Input: part model. Units: mm. Frame: model coordinates. Round coordinates to 2 decimals unless told otherwise and drop trailing zeros. Loops run counter-clockwise (first coordinate to the right, second up) from the corner with the lowest first, then second, coordinate; pieces in that order, holes last. Notation, with made-up numbers: (61.25, 85.5) - (118.25, 85.5) arc R26 ccw to (118.25, 124.5) - close; hole circle Ø11 at (-26.5, 80). An arc over 180 degrees is marked (long way). Use CSV: the item, a comma, the result in double quotes. Start each with the question number.
1. Cut plane A-A (x = 0.1). Return loops of the section in (y, z).
2. Material intervals for probe 1 along Y at (x, z) = (0.15, -0.75); probe 2 along Y at (x, z) = (-0.2, 5); probe 3 along Z at (x, y) = (0.1, 2), sorted ascending. Write a range as from..to.
3. Cut plane D-D (z = 4.5). Return loops of the section in (x, y), and give its area (3 significant figures).
4. Cut plane B-B (z = 2). Return loops of the section in (x, y), and give its area (3 significant figures).
5. Cut plane C-C (y = 0). Return loops of the section in (x, z).
```python
from build123d import *

# Parameters (mm, degrees)
BOSS_EXTRUDE1_DEPTH      = 0.3175
BOSS_EXTRUDE1_DEPTH_BACK = 0.3175
FILLET1_R                = 0.4445
FILLET2_R                = 0.22225


with BuildPart() as part:
    # Sketch3 → Boss-Extrude1 (new body, two sides)
    with BuildSketch(Plane(origin=(0, 0, 0), x_dir=(0, 0, -1), z_dir=(1, 0, 0))) as boss_extrude1_sk:
        with BuildLine():
            Line((2.493993522, -0.831331174), (4.564354048, -1.521451349))
            ThreePointArc((4.564354048, -1.521451349), (2.8131883, -3.903090272), (0, -4.811251613))
            Line((0, -4.811251613), (0, -2.6289))
            ThreePointArc((0, -2.6289), (-0.831331174, -2.493993522), (-1.57734, -2.10312))
            Line((-1.57734, -2.10312), (-5.759367109, -3.409486899))
            ThreePointArc((-5.759367109, -3.409486899), (6.6929, 0), (-5.759367109, 3.409486899))
            Line((-5.759367109, 3.409486899), (-1.57734, 2.10312))
            ThreePointArc((-1.57734, 2.10312), (-0.831331174, 2.493993522), (0, 2.6289))
            Line((0, 2.6289), (0, 4.811251613))
            ThreePointArc((0, 4.811251613), (2.8131883, 3.903090272), (4.564354048, 1.521451349))
            Line((4.564354048, 1.521451349), (2.493993522, 0.831331174))
            ThreePointArc((2.493993522, 0.831331174), (2.6289, 0), (2.493993522, -0.831331174))
        make_face()
    extrude(amount=BOSS_EXTRUDE1_DEPTH)
    extrude(boss_extrude1_sk.sketch, amount=-BOSS_EXTRUDE1_DEPTH_BACK)

    # Fillet1
    fillet1_edges = [part.edges().sort_by_distance(p)[0] for p in [
        (0, 1.521451349, -4.564354048),
        (0, 4.811251613, 0),
        (0, 3.409486899, 5.759367109),
        (0, -3.409486899, 5.759367109),
        (0, -4.811251613, 0),
        (0, -1.521451349, -4.564354048),
    ]]
    fillet(fillet1_edges, radius=FILLET1_R)

    # Fillet2
    fillet2_edges = [part.edges().sort_by_distance(p)[0] for p in [
        (0, 0.831331174, -2.493993522),
        (0, 2.6289, 0),
        (0, 2.10312, 1.57734),
        (0, -2.10312, 1.57734),
        (0, -2.6289, 0),
        (0, -0.831331174, -2.493993522),
    ]]
    fillet(fillet2_edges, radius=FILLET2_R)


solid = part.part
```
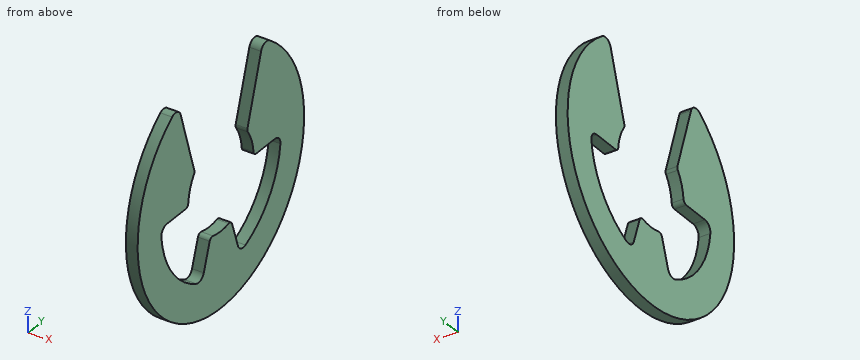
Established:
1,outline,"(-4.79, -0.49) arc R0.44 cw to (-4.34, 0) - (-2.84, 0) arc R0.22 ccw to (-2.62, 0.2) arc R2.63 cw to (-2.17, 1.49) arc R0.22 ccw to (-2.14, 1.68) - (-3.23, 5.2) arc R0.44 ccw to (-3.92, 5.43) arc R6.69 ccw (long way) to (3.92, 5.43) arc R0.44 ccw to (3.23, 5.2) - (2.14, 1.68) arc R0.22 ccw to (2.17, 1.49) arc R2.63 cw to (2.62, 0.2) arc R0.22 ccw to (2.84, 0) - (4.34, 0) arc R0.44 cw to (4.79, -0.49) arc R4.81 cw to (1.98, -4.39) arc R0.44 cw to (1.37, -4.12) - (0.9, -2.7) arc R0.22 ccw to (0.63, -2.55) arc R2.63 cw to (-0.63, -2.55) arc R0.22 ccw to (-0.9, -2.7) - (-1.37, -4.12) arc R0.44 cw to (-1.98, -4.39) arc R4.81 cw to start"
2,probe 1,"y = -6.65..-4.75, 4.75..6.65"
2,probe 2,"y = -4.45..-3.17, 3.17..4.45"
2,probe 3,"z = -6.39..-4.38"
3,outline,"(-0.32, -4.95) - (0.32, -4.95) - (0.32, -3.02) - (-0.32, -3.02) - close; (-0.32, 3.02) - (0.32, 3.02) - (0.32, 4.95) - (-0.32, 4.95) - close"
3,area,"2.46 mm2"
4,outline,"(-0.32, -6.39) - (0.32, -6.39) - (0.32, -2.24) - (-0.32, -2.24) - close; (-0.32, 2.24) - (0.32, 2.24) - (0.32, 6.39) - (-0.32, 6.39) - close"
4,area,"5.27 mm2"
5,outline,"(-0.32, -6.69) - (0.32, -6.69) - (0.32, -2.63) - (-0.32, -2.63) - close"
